Build history of the part. All positions in model axes, mm. A direction names the side the tool comes from. Coordinates: 2 decimals unless noted, no trailing zeros. Order: outer loops, then holes, each group sorted by start corner. A loop starts at its lowest first (then second) coordinate and runs counter-clockwise, first axis right, second up. Notation, with made-up numbers: (-21, 61.5) - (-17, 61.5) arc R35 ccw to (-17, 99.5) - close; hole circle Ø11 at (18.25, -16.5). An arc over 180 degrees is marked (long way). Return JSON: item names as keys, results as strings.
from build123d import *

# Parameters (mm, degrees)
F0_W     = 38.1
F0_H     = 76.2
F1_DEPTH = 15.24
F2_W     = 30.48
F2_H     = 12.7
F3_DEPTH = 12.7


with BuildPart() as f1:
    # F0 (on Front) → F1 (new body)
    with BuildSketch(Plane.XZ):
        with Locations((19.05, 38.1)):
            Rectangle(F0_W, F0_H)
    extrude(amount=F1_DEPTH)

    # F2 (on face) → F3 (cut)
    with BuildSketch(Plane.XZ.offset(15.24)):
        with Locations((18.9144, 47.031553)):
            Rectangle(F2_W, F2_H)
        with Locations((18.9144, 29.099608)):
            Rectangle(F2_W, F2_H)
        with Locations((18.9144, 10.842167)):
            Rectangle(F2_W, F2_H)
        with Locations((18.84441, 64.723954)):
            Rectangle(F2_W, F2_H)
    extrude(amount=-F3_DEPTH, mode=Mode.SUBTRACT)


solid = f1.part
1. Mould opens along X. For faces 1 (the flat face through (19, -9, 17.192)), 2 (the flat face through (0, -8, 38)), 3 (the flat face through (19, 0, 39)) say: pulls with the +X half, pulls with the -X half, needs draft (parallel to the pull), parting line crosses it, or undercut.
Check values:
{"face 1": "undercut", "face 2": "pulls with the -X half", "face 3": "needs draft"}
2. Tool access for faces 4 (the flat face through (3.674, -9, 29)), 5 (the flat face through (38.1, -8, 38)): list every direction of +Z, -Z, +X, -X, +Y, -Y with a clear straight run to the whole face (end or side of a thin tool).
Check values:
{"face 4": "-Y", "face 5": "+Z, -Z, +X, +Y, -Y"}
3. Probe L1, parallel to Z at x = 22, y = -5.75; L2, parallel to X at y = -7.75, z = 14; L3, parallel to X at y = -12.5, z = 66. List the from-to ranges inside material, lowest first.
Check values:
{"L1": "0 to 4.49, 17.19 to 22.75, 35.45 to 40.68, 53.38 to 58.37, 71.07 to 76.2", "L2": "0 to 3.67, 34.15 to 38.1", "L3": "0 to 3.6, 34.08 to 38.1"}
4. Cut at C-C on z = 65.5. Give the cut face in (x, y), plus the area to 3 significant figures.
Check values:
{"outline": "(0, -15.24) - (3.6, -15.24) - (3.6, -2.54) - (34.08, -2.54) - (34.08, -15.24) - (38.1, -15.24) - (38.1, 0) - (0, 0) - close", "area": "194 mm²"}
5. Cut at A-A on x = 16. Give the cut face in (y, z).
Check values:
{"outline": "(-15.24, 0) - (0, 0) - (0, 76.2) - (-15.24, 76.2) - (-15.24, 71.07) - (-2.54, 71.07) - (-2.54, 58.37) - (-15.24, 58.37) - (-15.24, 53.38) - (-2.54, 53.38) - (-2.54, 40.68) - (-15.24, 40.68) - (-15.24, 35.45) - (-2.54, 35.45) - (-2.54, 22.75) - (-15.24, 22.75) - (-15.24, 17.19) - (-2.54, 17.19) - (-2.54, 4.49) - (-15.24, 4.49) - close"}
6. Cut at B-B on y = -7.25. Give the cut face in (x, z).
Check values:
{"outline": "(0, 0) - (38.1, 0) - (38.1, 76.2) - (0, 76.2) - close; hole (3.6, 58.37) - (34.08, 58.37) - (34.08, 71.07) - (3.6, 71.07) - close; hole (3.67, 4.49) - (34.15, 4.49) - (34.15, 17.19) - (3.67, 17.19) - close; hole (3.67, 22.75) - (34.15, 22.75) - (34.15, 35.45) - (3.67, 35.45) - close; hole (3.67, 40.68) - (34.15, 40.68) - (34.15, 53.38) - (3.67, 53.38) - close"}
